Can you work these out from the model? Positions are in its coordinate system, mm. A direction names the side the tool comes from. Give positions to 0.01 mm unless a question says otherwise; leave off trailing zeros. Write each loop counter-clockwise with the first axis right and the second up, starting at its lowest first coordinate (ties: lowest second). Pieces come first, ordered by that corner, then holes.
```python
from build123d import *

# Parameters (mm, degrees)
SKETCH1_W           = 25.2
SKETCH1_H           = 24.9
SKETCH1_R           = 3.9
BOSS_EXTRUDE5_DEPTH = 1.8
SKETCH1_3_W         = 33.6
SKETCH1_3_H         = 33.6
SKETCH1_3_W_2       = 25.2
SKETCH1_3_H_2       = 24.9
BOSS_EXTRUDE6_DEPTH = 10
FILLET1_R           = 5
SKETCH3_W           = 18
SKETCH3_H           = 6.7
CUT_EXTRUDE1_DEPTH  = 3.8


with BuildPart() as part:
    # Sketch1 → Boss-Extrude5 (new body)
    with BuildSketch(Plane.XY):
        with Locations((-0.721052632, -0.003756028)):
            Rectangle(SKETCH1_W, SKETCH1_H)
        with Locations((-0.721052632, -2.353756028)):
            Circle(SKETCH1_R, mode=Mode.SUBTRACT)
    extrude(amount=-BOSS_EXTRUDE5_DEPTH)

    # Sketch1<3> → Boss-Extrude6 (add)
    with BuildSketch(Plane.XY):
        with Locations((-0.721052632, -2.353756028)):
            Rectangle(SKETCH1_3_W, SKETCH1_3_H)
        with Locations((-0.721052632, -0.003756028)):
            Rectangle(SKETCH1_3_W_2, SKETCH1_3_H_2, mode=Mode.SUBTRACT)
    extrude(amount=-BOSS_EXTRUDE6_DEPTH)

    # Fillet1
    fillet1_edges = [part.edges().sort_by_distance(p)[0] for p in [
        (16.078947368, 14.446243972, -5),
        (16.078947368, -19.153756028, -5),
        (-17.521052632, -19.153756028, -5),
        (-17.521052632, 14.446243972, -5),
    ]]
    fillet(fillet1_edges, radius=FILLET1_R)

    # Sketch3 → Cut-Extrude1 (cut)
    with BuildSketch(Plane(origin=(0, 0, -10), x_dir=(-1, 0, 0), z_dir=(0, 0, -1))):
        with Locations((0.721052632, -15.803756028)):
            Rectangle(SKETCH3_W, SKETCH3_H)
    extrude(amount=-CUT_EXTRUDE1_DEPTH, mode=Mode.SUBTRACT)


solid = part.part
```
1) Suppose I cut it at B-B on x = 9. Write out the boundary of the cut face in (y, z).
Values follow:
outline: (-19.15, -10) - (-12.45, -10) - (-12.45, -1.8) - (12.45, -1.8) - (12.45, -10) - (14.45, -10) - (14.45, 0) - (-19.15, 0) - close
2) Please list where these lines run through material, in increasing order: L1, parallel to Y at x = -7.5, z = -5.75; L2, parallel to X at y = -7, z = -7.75; L3, parallel to Z at x = -5, y = -17.5.
Values follow:
L1: y = -19.15 to -12.45, 12.45 to 14.45
L2: x = -17.52 to -13.32, 11.88 to 16.08
L3: z = -6.2 to 0
3) For pin 1 Ø1.1 at (y, z) = (-15, -7.5) entering from -X; pin 2 Ø7.5 at (x, y) = (-0.5, -17) entering from -Z; pin 3 Ø8 at (x, y) = (-5, -5.5) entering from -Z, each with a flat end and sliding along its axis, tell me the tip position at first contact or that it passes through.
Values follow:
pin 1: stops at x = -17.51
pin 2: stops at z = -6.2
pin 3: stops at z = -1.8
4) Suppose I cut it at D-D on z = -7. Write out the boundary of the cut face in (x, y).
Values follow:
outline: (-17.52, -14.15) arc R5 ccw to (-12.52, -19.15) - (-9.72, -19.15) - (-9.72, -12.45) - (-13.32, -12.45) - (-13.32, 12.45) - (11.88, 12.45) - (11.88, -12.45) - (8.28, -12.45) - (8.28, -19.15) - (11.08, -19.15) arc R5 ccw to (16.08, -14.15) - (16.08, 9.45) arc R5 ccw to (11.08, 14.45) - (-12.52, 14.45) arc R5 ccw to (-17.52, 9.45) - close
5) Suppose I cut it at A-A on z = -3.75. Write out the boundary of the cut face in (x, y), plus the area to 3 significant figures.
Values follow:
outline: (-17.52, -14.15) arc R5 ccw to (-12.52, -19.15) - (11.08, -19.15) arc R5 ccw to (16.08, -14.15) - (16.08, 9.45) arc R5 ccw to (11.08, 14.45) - (-12.52, 14.45) arc R5 ccw to (-17.52, 9.45) - close; hole (-13.32, -12.45) - (11.88, -12.45) - (11.88, 12.45) - (-13.32, 12.45) - close
area: 480 mm2
6) Suppose I cut it at C-C on y = -3. Write out the boundary of the cut face in (x, z).
Values follow:
outline: (-17.52, -10) - (-13.32, -10) - (-13.32, -1.8) - (-4.57, -1.8) - (-4.57, 0) - (-17.52, 0) - close; (3.13, -1.8) - (11.88, -1.8) - (11.88, -10) - (16.08, -10) - (16.08, 0) - (3.13, 0) - close
7) For faces 1 (the face through (-1, -12.454, -5)), 2 (the face through (-1, -16, -6.2)), 3 (the face through (14.575, 13.02, -5.07)), which set-ups out of +Z, -Z, +X, -X, +Y, -Y let a thin tool reach every point of the face, with its end or its side?
Values follow:
face 1: -Z
face 2: -Z, -Y
face 3: +Z, -Z, +X, +Y
8) If we mould it in two halves opening along X, with no side actions, what happens to faces 4 (the face through (-16.095, -17.65, -5.07)), 5 (the face through (-3, 13, -10)), 6 (the face through (14.575, -17.728, -5.07)), 7 (the face through (8.279, -16, -8))? For each: +X half, -X half, draft (parallel to the pull), parting line (faces both ways), or undercut.
Values follow:
face 4: -X half
face 5: draft
face 6: +X half
face 7: undercut
